Autodesk Inventor part; units mm, degrees
ref_plane "YZ Plane" through (0, 0, 0) normal (1, 0, 0) x (0, 1, 0)
ref_plane "XZ Plane" through (0, 0, 0) normal (0, 1, 0) x (-1, 0, 0)
ref_plane "XY Plane" through (0, 0, 0) normal (0, 0, 1) x (1, 0, 0)
sketch "スケッチ1" plane through (0, 0, 0) normal (0, 0, 1) x (1, 0, 0)
  circle A0 centre (0, 0) radius 1.5
  dimension "d0" = 3
extrude "押し出し1" add sketch "スケッチ1" along normal blind 5
sketch "スケッチ2" plane through (0, 0, 0) normal (0, 0, -1) x (-1, 0, 0)
  circle A0 centre (0, 0) radius 3
  dimension "d3" = 6
extrude "押し出し2" add sketch "スケッチ2" against normal blind 2
thread "ねじ1"
chamfer "面取り1" distance 1.5 angle 45 1 edges at (3, 0, 2)
properties part number "ネジ皿m3,05" material "鋼、高強度、低合金"
Can you work these out from the model? Positions are in its coordinate system, mm. A direction names the side the tool comes from. Round coordinates to 2 decimals unless told otherwise and drop trailing zeros. Loops run counter-clockwise (first coordinate to the right, second up) from the corner with the lowest first, then second, coordinate; pieces in that order, holes last. Notation, with made-up numbers: M -5.75,35.25 L 4.25,35.25 A25 ccw 4.25,72.25 Z; hole C 5,-30 d1. An arc over 180 degrees is marked long. Write item = value, one per line. Start each with the question number.
(1) Suppose I cut it at D-D on z = 0.65. Write out the boundary of the cut face in (x, y).
(2) Which directions (+Z, -Z, +X, -X, +Y, -Y) give clear straight access to the entire face, cutting with the end or side of a thin tool? Please do faces 1 (the face through (3, 0.1, 0.2)), 2 (the face through (-1.5, -0.07, 3.48)).
(3) Suppose I cut it at C-C on z = 2.1. Write out the boundary of the cut face in (x, y), plus the area to 3 significant figures.
(4) I need wall thicknesses on line 1 along Z through (x, y) = (2, -0.05); line 2 along Y through (x, z) = (0.05, 3.45); line 3 along X through (y, z) = (1.6, 0.35). Which ranges of each line are inside material? Lowest first, please.
(5) I'm going to push flat-ended pins straight in: P1, Ø1, axis at x = 2.5, y = -1.5, coming from the +Z side; P2, Ø3, axis at x = 2, z = 2, coming from the -Y side; P3, Ø2, axis at x = 1.5, z = 4.5, coming from the +Y side. Where does each tip first touch, or does it pass through?
Answer block:
q1.outline = C 0,0 d5.7
q2.face_1 = +Z, -Z
q2.face_2 = +Z
q3.outline = C 0,0 d3
q3.area = 7.07 mm²
q4.line_1 = 0 to 1.5
q4.line_2 = -1.5 to 1.5
q4.line_3 = -2.54 to 2.54
q5.P1 = 1.08
q5.P2 = -2.51
q5.P3 = 1.41
